Source: CAD feature listing. Evaluate the final solid. Frame: model axes, mm. A direction names the side the tool comes from. Give positions to 0.01 mm unless a question says otherwise; leave off trailing zeros. Order: outer loops, then holes, each group sorted by start corner. A loop starts at its lowest first (then second) coordinate and runs counter-clockwise, first axis right, second up.
from build123d import *

# Parameters (mm, degrees)
SKETCH_1_W               = 19.8
SKETCH_1_H               = 10
EXTRUDE_1_DEPTH          = 6.9
SKETCH_2_W               = 0.6
SKETCH_2_H               = 0.2
PATTERN_LINEAR_1_COUNT   = 4
PATTERN_LINEAR_1_PITCH   = 2.54
MIRROR_1_COPY_1_SKETCH_W = 0.6
MIRROR_1_COPY_1_SKETCH_H = 0.2
MIRROR_1_COPY_2_SKETCH_W = 0.6
MIRROR_1_COPY_2_SKETCH_H = 0.2
MIRROR_1_COPY_3_SKETCH_W = 0.6
MIRROR_1_COPY_3_SKETCH_H = 0.2
SKETCH_5_W               = 0.6
SKETCH_5_H               = 0.2
PATTERN_LINEAR_2_COUNT   = 4
PATTERN_LINEAR_2_PITCH   = 2.54
MIRROR_2_COPY_1_SKETCH_W = 0.6
MIRROR_2_COPY_1_SKETCH_H = 0.2
MIRROR_2_COPY_2_SKETCH_W = 0.6
MIRROR_2_COPY_2_SKETCH_H = 0.2
MIRROR_2_COPY_3_SKETCH_W = 0.6
MIRROR_2_COPY_3_SKETCH_H = 0.2
SKETCH_7_W               = 0.71
SKETCH_7_H               = 0.4
SKETCH_7_W_2             = 1.94
CUT_EXTRUDE_1_DEPTH      = 24.230368056
SKETCH_8_W               = 0.4
SKETCH_8_H               = 3.904109304
SKETCH_8_H_2             = 5.232387761
CUT_EXTRUDE_2_DEPTH      = 24.230368056


with BuildPart() as part:
    # Sketch 1 → Extrude 1 (new body)
    with BuildSketch(Plane.XY):
        with Locations((9.9, 5)):
            Rectangle(SKETCH_1_W, SKETCH_1_H)
    extrude(amount=EXTRUDE_1_DEPTH)

    # Sweep 2: sweep along a path in Sketch 3
    with BuildLine(Plane(origin=(11.17, 0, 0), x_dir=(0, 0, -1), z_dir=(1, 0, 0))) as sweep_2_path:
        Line((0, 2.022879956), (0.5, 2.022879956))
        Line((0.5, 2.022879956), (0.5, -1.8))
    # Sketch 2 → Sweep 2 (sweep)
    with BuildSketch(Plane(origin=(0, 0, 0), x_dir=(-1, 0, 0), z_dir=(0, 0, -1))):
        with Locations((-11.17, 1.72257922)):
            Rectangle(SKETCH_2_W, SKETCH_2_H)
    sweep_2 = sweep(path=sweep_2_path.line, transition=Transition.RIGHT)

    # Pattern Linear 1: Sweep 2 ×4
    with Locations(*[(i * PATTERN_LINEAR_1_PITCH, 0, 0) for i in range(1, PATTERN_LINEAR_1_COUNT)]):
        add(sweep_2)

    # Mirror 1: Sweep 2 across plane
    add(sweep_2.mirror(Plane(origin=(9.9, 0, 0), x_dir=(0, 0, 1), z_dir=(1, 0, 0))))

    # Mirror 1 copy 1: sweep along a path in Mirror 1 copy 1 path
    with BuildLine(Plane(origin=(6.09, 0, 0), x_dir=(0, 0, -1), z_dir=(-1, 0, 0))) as mirror_1_copy_1_path:
        Line((0, -2.022879956), (0.5, -2.022879956))
        Line((0.5, -2.022879956), (0.5, 1.8))
    # Mirror 1 copy 1 sketch → Mirror 1 copy 1 (sweep)
    with BuildSketch(Plane(origin=(17.26, 0, 0), x_dir=(1, 0, 0), z_dir=(0, 0, -1))):
        with Locations((-11.17, -1.72257922)):
            Rectangle(MIRROR_1_COPY_1_SKETCH_W, MIRROR_1_COPY_1_SKETCH_H)
    sweep(path=mirror_1_copy_1_path.line, transition=Transition.RIGHT)

    # Mirror 1 copy 2: sweep along a path in Mirror 1 copy 2 path
    with BuildLine(Plane(origin=(3.55, 0, 0), x_dir=(0, 0, -1), z_dir=(-1, 0, 0))) as mirror_1_copy_2_path:
        Line((0, -2.022879956), (0.5, -2.022879956))
        Line((0.5, -2.022879956), (0.5, 1.8))
    # Mirror 1 copy 2 sketch → Mirror 1 copy 2 (sweep)
    with BuildSketch(Plane(origin=(14.72, 0, 0), x_dir=(1, 0, 0), z_dir=(0, 0, -1))):
        with Locations((-11.17, -1.72257922)):
            Rectangle(MIRROR_1_COPY_2_SKETCH_W, MIRROR_1_COPY_2_SKETCH_H)
    sweep(path=mirror_1_copy_2_path.line, transition=Transition.RIGHT)

    # Mirror 1 copy 3: sweep along a path in Mirror 1 copy 3 path
    with BuildLine(Plane(origin=(1.01, 0, 0), x_dir=(0, 0, -1), z_dir=(-1, 0, 0))) as mirror_1_copy_3_path:
        Line((0, -2.022879956), (0.5, -2.022879956))
        Line((0.5, -2.022879956), (0.5, 1.8))
    # Mirror 1 copy 3 sketch → Mirror 1 copy 3 (sweep)
    with BuildSketch(Plane(origin=(12.18, 0, 0), x_dir=(1, 0, 0), z_dir=(0, 0, -1))):
        with Locations((-11.17, -1.72257922)):
            Rectangle(MIRROR_1_COPY_3_SKETCH_W, MIRROR_1_COPY_3_SKETCH_H)
    sweep(path=mirror_1_copy_3_path.line, transition=Transition.RIGHT)

    # Sweep 3: sweep along a path in Sketch 6
    with BuildLine(Plane(origin=(11.17, 0, 0), x_dir=(0, 0, -1), z_dir=(1, 0, 0))) as sweep_3_path:
        Line((0, 7.391909702), (2.839699264, 7.391909702))
        Line((2.839699264, 7.391909702), (2.839699264, -1.8))
    # Sketch 5 → Sweep 3 (sweep)
    with BuildSketch(Plane(origin=(0, 0, 0), x_dir=(-1, 0, 0), z_dir=(0, 0, -1))):
        with Locations((-11.17, 7.291909702)):
            Rectangle(SKETCH_5_W, SKETCH_5_H)
    sweep_3 = sweep(path=sweep_3_path.line, transition=Transition.RIGHT)

    # Pattern Linear 2: Sweep 3 ×4
    with Locations(*[(i * PATTERN_LINEAR_2_PITCH, 0, 0) for i in range(1, PATTERN_LINEAR_2_COUNT)]):
        add(sweep_3)

    # Mirror 2: Sweep 3 across plane
    add(sweep_3.mirror(Plane(origin=(9.9, 0, 0), x_dir=(0, 0, 1), z_dir=(1, 0, 0))))

    # Mirror 2 copy 1: sweep along a path in Mirror 2 copy 1 path
    with BuildLine(Plane(origin=(6.09, 0, 0), x_dir=(0, 0, -1), z_dir=(-1, 0, 0))) as mirror_2_copy_1_path:
        Line((0, -7.391909702), (2.839699264, -7.391909702))
        Line((2.839699264, -7.391909702), (2.839699264, 1.8))
    # Mirror 2 copy 1 sketch → Mirror 2 copy 1 (sweep)
    with BuildSketch(Plane(origin=(17.26, 0, 0), x_dir=(1, 0, 0), z_dir=(0, 0, -1))):
        with Locations((-11.17, -7.291909702)):
            Rectangle(MIRROR_2_COPY_1_SKETCH_W, MIRROR_2_COPY_1_SKETCH_H)
    sweep(path=mirror_2_copy_1_path.line, transition=Transition.RIGHT)

    # Mirror 2 copy 2: sweep along a path in Mirror 2 copy 2 path
    with BuildLine(Plane(origin=(3.55, 0, 0), x_dir=(0, 0, -1), z_dir=(-1, 0, 0))) as mirror_2_copy_2_path:
        Line((0, -7.391909702), (2.839699264, -7.391909702))
        Line((2.839699264, -7.391909702), (2.839699264, 1.8))
    # Mirror 2 copy 2 sketch → Mirror 2 copy 2 (sweep)
    with BuildSketch(Plane(origin=(14.72, 0, 0), x_dir=(1, 0, 0), z_dir=(0, 0, -1))):
        with Locations((-11.17, -7.291909702)):
            Rectangle(MIRROR_2_COPY_2_SKETCH_W, MIRROR_2_COPY_2_SKETCH_H)
    sweep(path=mirror_2_copy_2_path.line, transition=Transition.RIGHT)

    # Mirror 2 copy 3: sweep along a path in Mirror 2 copy 3 path
    with BuildLine(Plane(origin=(1.01, 0, 0), x_dir=(0, 0, -1), z_dir=(-1, 0, 0))) as mirror_2_copy_3_path:
        Line((0, -7.391909702), (2.839699264, -7.391909702))
        Line((2.839699264, -7.391909702), (2.839699264, 1.8))
    # Mirror 2 copy 3 sketch → Mirror 2 copy 3 (sweep)
    with BuildSketch(Plane(origin=(12.18, 0, 0), x_dir=(1, 0, 0), z_dir=(0, 0, -1))):
        with Locations((-11.17, -7.291909702)):
            Rectangle(MIRROR_2_COPY_3_SKETCH_W, MIRROR_2_COPY_3_SKETCH_H)
    sweep(path=mirror_2_copy_3_path.line, transition=Transition.RIGHT)

    # Sketch 7 → Cut-Extrude 1 (cut, through all)
    with BuildSketch(Plane.XZ):
        with Locations((0.355, 6.7)):
            Rectangle(SKETCH_7_W, SKETCH_7_H)
        with Locations((2.28, 6.7)):
            Rectangle(SKETCH_7_W_2, SKETCH_7_H)
        with Locations((4.82, 6.7)):
            Rectangle(SKETCH_7_W_2, SKETCH_7_H)
        with Locations((9.9, 6.7)):
            Rectangle(SKETCH_7_W_2, SKETCH_7_H)
        with Locations((7.36, 6.7)):
            Rectangle(SKETCH_7_W_2, SKETCH_7_H)
        with Locations((12.44, 6.7)):
            Rectangle(SKETCH_7_W_2, SKETCH_7_H)
        with Locations((14.98, 6.7)):
            Rectangle(SKETCH_7_W_2, SKETCH_7_H)
        with Locations((17.52, 6.7)):
            Rectangle(SKETCH_7_W_2, SKETCH_7_H)
        with Locations((19.445, 6.7)):
            Rectangle(SKETCH_7_W, SKETCH_7_H)
    extrude(amount=-CUT_EXTRUDE_1_DEPTH, mode=Mode.SUBTRACT)

    # Sketch 8 → Cut-Extrude 2 (cut, through all)
    with BuildSketch(Plane(origin=(19.8, 0, 0), x_dir=(0, 0, -1), z_dir=(1, 0, 0))):
        with Locations((-6.7, 8.047945348)):
            Rectangle(SKETCH_8_W, SKETCH_8_H)
        with Locations((-6.7, 2.616193881)):
            Rectangle(SKETCH_8_W, SKETCH_8_H_2)
    extrude(amount=-CUT_EXTRUDE_2_DEPTH, mode=Mode.SUBTRACT)


solid = part.part
1) Section query A-A on z = -1.5. State how many separate pieces and enclosed holes the cut face has, and give its area (3 significant figures).
Checks:
separate pieces: 8
enclosed holes: 0
area: 0.960 mm2
2) Ray query, L1, parallel to Z at x = 16.5, y = 2; L2, parallel to Z at x = 5.5, y = 7; L3, parallel to Y at x = 18.75, z = -0.75. Return the intervals inside material, ascending.
Checks:
L1: z = -2.84 to -2.64, 0 to 6.5
L2: z = 0 to 6.5
L3: y = 7.19 to 7.39
3) First-contact query: pin 1 Ø0.7 at (x, z) = (11, -1.5) entering from +Y; pin 2 Ø0.7 at (x, y) = (18.5, 1.5) entering from +Z. Flat tips, straight axial feed; report the tip coordinate or a pass-through.
Checks:
pin 1: stops at y = 7.39
pin 2: stops at z = 6.5
4) Reachability of faces 1 (the face through (0, 5, 3)), 2 (the face through (10, 0, 3)) from +Z, -Z, +X, -X, +Y, -Y: full face, straight path, thin tool, end or side. Return the list, or none.
Checks:
face 1: +Z, -Z, -X, +Y, -Y
face 2: +Z, +X, -X, -Y
5) Section query D-D on z = 2.25. Output: boundary loops of the cut face in (x, y).
Checks:
outline: (0, 0) - (19.8, 0) - (19.8, 10) - (0, 10) - close
